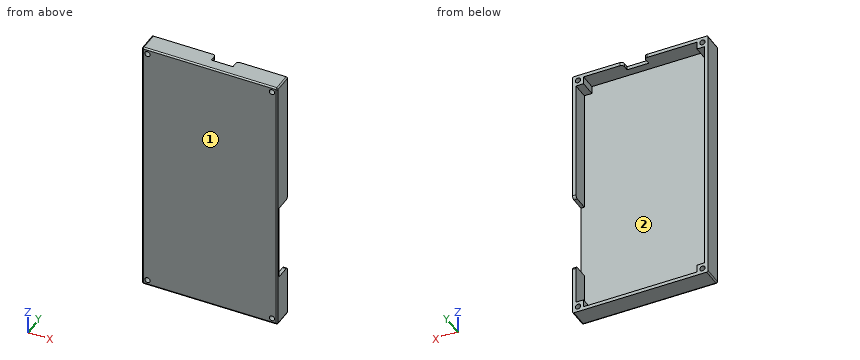
Autodesk Inventor part; units mm, degrees
ref_plane "YZ Plane" through (0, 0, 0) normal (1, 0, 0) x (0, 1, 0)
ref_plane "XZ Plane" through (0, 0, 0) normal (0, 1, 0) x (-1, 0, 0)
ref_plane "XY Plane" through (0, 0, 0) normal (0, 0, 1) x (1, 0, 0)
sketch "Sketch1" plane through (0, 0, 0) normal (0, 1, 0) x (-1, 0, 0)
  line L0 (0, 0) -> (62.23, 0)
  line L1 (62.23, 0) -> (62.23, -120.65)
  line L2 (62.23, -120.65) -> (0, -120.65)
  line L3 (0, -120.65) -> (0, 0)
  dimension "d0" = 62.23
  dimension "d1" = 120.65
extrude "Extrusion1" add sketch "Sketch1" along normal blind 1.5
sketch "Sketch2" plane through (0, 1.5, 0) normal (0, 1, 0) x (1, 0, 0)
  line L0 (-60.6425, 1.5875) -> (-1.5875, 1.5875)
  line L1 (-1.5875, 1.5875) -> (-1.5875, 119.0625)
  line L2 (-1.5875, 119.0625) -> (-60.6425, 119.0625)
  line L3 (-60.6425, 119.0625) -> (-60.6425, 1.5875)
  line L4 (-62.23, 0) -> (0, 0)
  line L5 (0, 0) -> (0, 120.65)
  line L6 (-62.23, 120.65) -> (-62.23, 0)
  line L7 (0, 120.65) -> (-62.23, 120.65)
  line L8 (0, 0) -> (-5.08, 0)
  line L9 (-5.08, 0) -> (-5.08, 5.08)
  line L10 (-5.08, 5.08) -> (0, 5.08)
  line L11 (0, 5.08) -> (0, 0)
  line L12 (-62.23, 0) -> (-57.15, 0)
  line L13 (-57.15, 0) -> (-57.15, 5.08)
  line L14 (-57.15, 5.08) -> (-62.23, 5.08)
  line L15 (-62.23, 5.08) -> (-62.23, 0)
  line L16 (0, 120.65) -> (-5.08, 120.65)
  line L17 (-5.08, 120.65) -> (-5.08, 115.57)
  line L18 (-5.08, 115.57) -> (0, 115.57)
  line L19 (0, 115.57) -> (0, 120.65)
  line L20 (-62.23, 120.65) -> (-57.15, 120.65)
  line L21 (-57.15, 120.65) -> (-57.15, 115.57)
  line L22 (-57.15, 115.57) -> (-62.23, 115.57)
  line L23 (-62.23, 115.57) -> (-62.23, 120.65)
  point P0 (0, 115.57)
  point P1 (-1.5875, 115.57)
  point P2 (-1.5875, 5.08)
  point P3 (-5.08, 1.5875)
  point P4 (-57.15, 1.5875)
  point P5 (-60.6425, 5.08)
  point P6 (-5.08, 119.0625)
  point P7 (-60.6425, 115.57)
  point P8 (-57.15, 119.0625)
  dimension "d4" = 1.5875
  dimension "d5" = 1.5875
  dimension "d6" = 1.5875
  dimension "d7" = 1.5875
  dimension "d8" = 5.08
  dimension "d9" = 5.08
  dimension "d10" = 5.08
  dimension "d11" = 5.08
  dimension "d12" = 5.08
  dimension "d13" = 5.08
  dimension "d14" = 5.08
  dimension "d15" = 5.08
extrude "Extrusion3" add sketch "Sketch2" along normal blind 7.5 contours L3 L14 L13 L0 | L0 L13 L4 L6 L14 L3 | L0 L9 L4 L13 | L14 L6 L22 L3 | L9 L10 L1 L0 | L0 L1 L10 L5 L4 L9 | L22 L6 L7 L21 L2 L3 | L3 L2 L21 L22 | L1 L18 L5 L10 | L21 L7 L17 L2 | L18 L17 L2 L1 | L1 L2 L17 L7 L5 L18
sketch "Sketch3" plane through (0, 9, 0) normal (0, 1, 0) x (1, 0, 0)
  line L0 (-62.23, 0) -> (0, 0)
  line L1 (-33.02, 0) -> (-23.114, 0)
  line L2 (-23.114, 0) -> (-23.114, 1.5875)
  line L3 (-23.114, 1.5875) -> (-33.02, 1.5875)
  line L4 (-33.02, 1.5875) -> (-33.02, 0)
  line L5 (0, 0) -> (0, 120.65)
  line L6 (-62.23, 120.65) -> (-62.23, 0)
  line L7 (0, 120.65) -> (-62.23, 120.65)
  line L8 (-60.6425, 115.57) -> (-60.6425, 5.08)
  line L9 (-62.23, 60.325) -> (-60.6425, 60.325)
  line L10 (-60.6425, 60.325) -> (-60.6425, 98.425)
  line L11 (-60.6425, 98.425) -> (-62.23, 98.425)
  line L12 (-62.23, 98.425) -> (-62.23, 60.325)
  point P0 (-59.69, 2.54)
  point P1 (-59.69, 118.11)
  point P2 (-2.54, 118.11)
  point P3 (-2.54, 2.54)
  dimension "d20" = 23.114
  dimension "d22" = 2.54
  dimension "d23" = 2.54
  dimension "d24" = 2.54
  dimension "d25" = 2.54
  dimension "d26" = 2.54
  dimension "d27" = 2.54
  dimension "d28" = 2.54
  dimension "d29" = 2.54
  dimension "d47" = 60.325
  dimension "d48" = 22.225
  dimension "d59" = 33.02
extrude "Extrusion4" cut sketch "Sketch3" against normal blind 3.81 contours L4 L3 L2 L0
sketch "Sketch4" plane through (0, 9, 0) normal (0, 1, 0) x (1, 0, 0)
  line L0 (-23.114, 0) -> (0, 0)
  line L1 (0, 0) -> (0, 120.65)
  line L2 (-62.23, 0) -> (-33.02, 0)
  line L3 (-62.23, 120.65) -> (-62.23, 0)
  line L4 (0, 120.65) -> (-62.23, 120.65)
  point P0 (-2.54, 2.54)
  point P1 (-2.54, 118.11)
  point P2 (-59.69, 118.11)
  point P3 (-59.69, 2.54)
  dimension "d39" = 2.54
  dimension "d40" = 2.54
  dimension "d41" = 2.54
  dimension "d42" = 2.54
  dimension "d43" = 2.54
  dimension "d44" = 2.54
  dimension "d45" = 2.54
  dimension "d46" = 2.54
hole "Hole1" at (-2.54, 9, -2.54) at (-2.54, 9, -118.11) at (-59.69, 9, -118.11) at (-59.69, 9, -2.54) direction (0, -1, 0) diameter 2.4384 end through all
sketch "Sketch5" plane through (0, 9, 0) normal (0, 1, 0) x (1, 0, 0)
  line L0 (-62.23, 91.65) -> (-60.6425, 91.65)
  line L1 (-60.6425, 5.08) -> (-60.6425, 115.57)
  line L2 (-62.23, 120.65) -> (-62.23, 0)
  line L3 (-62.23, 79) -> (-60.6425, 79)
  line L4 (-62.23, 84) -> (-60.6425, 84)
  line L5 (-62.23, 75) -> (-60.6425, 75)
  line L6 (-62.23, 62) -> (-60.6425, 62)
  line L7 (-62.23, 0) -> (-33.02, 0)
  line L8 (0, 120.65) -> (-62.23, 120.65)
  line L9 (-62.23, 96.65) -> (-60.6425, 96.65)
  line L10 (-1.5875, 115.57) -> (-1.5875, 5.08)
  line L11 (-1.5875, 61.976) -> (0, 61.976)
  line L12 (-1.5875, 97.028) -> (0, 97.028)
  line L13 (0, 0) -> (0, 120.65)
  line L14 (-23.114, 0) -> (0, 0)
  dimension "d49" = 62
  dimension "d50" = 75
  dimension "d51" = 79
  dimension "d52" = 5
  dimension "d53" = 29
  dimension "d54" = 5
  dimension "d60" = 61.976
  dimension "d61" = 97.028
extrude "Extrusion5" cut sketch "Sketch5" against normal up to surface (7.5 mm away) contours L13 L11 L10 L12
fillet "Fillet1" radius 1.27 4 edges at (-33.02, 9, -0.7938) (-23.114, 9, -0.7938) (-0.7938, 9, -61.976) (-0.7938, 9, -97.028)
fillet "Fillet2" radius 0.635 8 edges at (-31.115, 0, 0) (0, 0, -60.325) (0, 4.5, 0) (-62.23, 4.5, 0) (-62.23, 0, -60.325) (-31.115, 0, -120.65) (0, 4.5, -120.65) (-62.23, 4.5, -120.65)
equation "\"d4\" = d5"
equation "\"d6\" = d5"
equation "\"d7\" = d5"
equation "\"d10\" = d8"
equation "\"d11\" = d10"
equation "\"d12\" = d8"
equation "\"d13\" = d8"
equation "\"d14\" = d8"
equation "\"d15\" = d8"
properties part number "cover_bottom"
Source: CAD feature listing. Evaluate the final solid. Frame: model axes, mm. Face numbers are marked on the shaded views. Round coordinates to 2 decimals unless told otherwise and drop trailing zeros. Loops run counter-clockwise (first coordinate to the right, second up) from the corner with the lowest first, then second, coordinate; pieces in that order, holes last. Notation, with made-up numbers: M -40,-14 L -34,-14 A17 ccw -34,-8 Z; hole C 31.5,87 d2. An arc over 180 degrees is marked long. Put each result on its own line as item: value.
(1) Section B-B, the plane z = -74.5. Return loops of the section in (x, y) (1 decimal).
Solutions:
outline: M -62.2,0.6 A0.6 ccw -61.6,0 L -0.6,0 A0.6 ccw 0,0.6 L 0,1.5 L -60.6,1.5 L -60.6,9 L -62.2,9 Z
(2) Section D-D, the plane z = -59.5. Return loops of the section in (x, y) (1 decimal), and give its area (3 significant figures).
Solutions:
outline: M -62.2,0.6 A0.6 ccw -61.6,0 L -0.6,0 A0.6 ccw 0,0.6 L 0,9 L -1.6,9 L -1.6,1.5 L -60.6,1.5 L -60.6,9 L -62.2,9 Z
area: 117 mm²
(3) Section A-A, the plane y = 2.75. State how many separate pieces and enclosed holes the cut face has, and give its area (3 significant figures).
Solutions:
separate pieces: 1
enclosed holes: 4
area: 545 mm²
(4) Ray query, line 1 (Z direction, x = -2.54, y = 2.5); line 2 (Z direction, x = -53.5, y = 6.25); line 3 (X direction, y = 4, z = -39). Return the intervals inside material, ascending. Write a range as [from, to].
Solutions:
line 1: [-120.65, -119.33], [-116.89, -115.57], [-5.08, -3.76], [-1.32, 0]
line 2: [-120.65, -119.06], [-1.59, 0]
line 3: [-62.23, -60.64], [-1.59, 0]
(5) Pull-direction query (Z, two-part tool) for the marked faces 1 and 2; classes: released by +Z, released by -Z, zero draft, split by the parting line, or undercut.
Solutions:
face 1: zero draft
face 2: undercut
